Work out the finished part from the listing and answer in its coordinate system (mm). Face numbers are marked on the shaded views. A direction names the side the tool comes from. Coordinates: 2 decimals unless noted, no trailing zeros. Order: outer loops, then holes, each group sorted by start corner. A loop starts at its lowest first (then second) coordinate and runs counter-clockwise, first axis right, second up. Notation, with made-up numbers: M 14,-14 L 32,-14 A16 cw 32,-8 Z; hole C 80.5,36.25 d4. An arc over 180 degrees is marked long. Use a Markdown table: item, result.
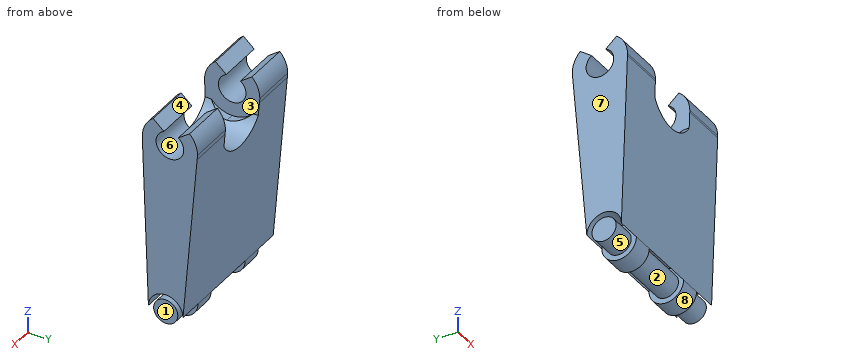
from build123d import *

# Parameters (mm, degrees)
SKETCH1_R           = 4
SKETCH1_R_2         = 5
SKETCH1_R_3         = 3.5
BOSS_EXTRUDE1_DEPTH = 21
SKETCH1_4_R         = 4
CUT_EXTRUDE2_DEPTH  = 8
SKETCH1_5_R         = 5
SKETCH1_5_R_2       = 3.5
CUT_EXTRUDE3_DEPTH  = 8
CUT_EXTRUDE4_START  = 21
SKETCH1_6_R         = 5
SKETCH1_6_R_2       = 3.5
CUT_EXTRUDE4_DEPTH  = 7
CUT_EXTRUDE5_DEPTH  = 10
CUT_EXTRUDE6_REACH  = 71.663


with BuildPart() as part:
    # Sketch1 → Boss-Extrude1 (new, symmetric)
    # profile 1 of 4: a face of its own
    with BuildSketch(Plane(origin=(0, 0, 0), x_dir=(0, 0, -1), z_dir=(1, 0, 0))):
        with BuildLine():
            Line((50, 3.790245356), (1.337639211, 7.887377342))
            ThreePointArc((1.337639211, 7.887377342), (6.111510193, 5.162309866), (8, 0))
            ThreePointArc((8, 0), (5.855645149, -5.450818277), (0.572145029, -7.9795144))
            Line((0.572145029, -7.9795144), (50, -6.209754644))
            ThreePointArc((50, -6.209754644), (45, -1.209754644), (50, 3.790245356))
        make_face()
    # profile 2 of 4: a face of its own
    with BuildSketch(Plane(origin=(0, 0, 0), x_dir=(0, 0, -1), z_dir=(1, 0, 0))):
        with BuildLine():
            Line((1.337639211, 7.887377342), (0, 8))
            ThreePointArc((0, 8), (-8, 0), (0, -8))
            Line((0, -8), (0.572145029, -7.9795144))
            ThreePointArc((0.572145029, -7.9795144), (5.855645149, -5.450818277), (8, 0))
            ThreePointArc((8, 0), (6.111510193, 5.162309866), (1.337639211, 7.887377342))
        make_face()
        with Locations(Location((0, 0, 0), (0, 0, 180))):
            Circle(SKETCH1_R, mode=Mode.SUBTRACT)
    # profile 3 of 4: a face of its own
    with BuildSketch(Plane(origin=(0, 0, 0), x_dir=(0, 0, -1), z_dir=(1, 0, 0))):
        with Locations((50, -1.209754644)):
            Circle(SKETCH1_R_2)
        with Locations((50, -1.209754644)):
            Circle(SKETCH1_R_3, mode=Mode.SUBTRACT)
    # profile 4 of 4: a face of its own
    with BuildSketch(Plane(origin=(0, 0, 0), x_dir=(0, 0, -1), z_dir=(1, 0, 0))):
        with Locations((50, -1.209754644)):
            Circle(SKETCH1_R_3)
    extrude(amount=BOSS_EXTRUDE1_DEPTH, both=True)

    # Sketch1<4> → Cut-Extrude2 (cut, symmetric)
    with BuildSketch(Plane(origin=(0, 0, 0), x_dir=(0, 0, -1), z_dir=(1, 0, 0))):
        with BuildLine():
            Line((1.337639211, 7.887377342), (0, 8))
            ThreePointArc((0, 8), (-8, 0), (0, -8))
            Line((0, -8), (0.572145029, -7.9795144))
            ThreePointArc((0.572145029, -7.9795144), (5.855645149, -5.450818277), (8, 0))
            ThreePointArc((8, 0), (6.111510193, 5.162309866), (1.337639211, 7.887377342))
        make_face()
        with Locations(Location((0, 0, 0), (0, 0, 180))):
            Circle(SKETCH1_4_R, mode=Mode.SUBTRACT)
    extrude(amount=CUT_EXTRUDE2_DEPTH, both=True, mode=Mode.SUBTRACT)

    # Sketch1<5> → Cut-Extrude3 (cut, symmetric)
    with BuildSketch(Plane(origin=(0, 0, 0), x_dir=(0, 0, -1), z_dir=(1, 0, 0))):
        with Locations((50, -1.209754644)):
            Circle(SKETCH1_5_R)
        with Locations((50, -1.209754644)):
            Circle(SKETCH1_5_R_2, mode=Mode.SUBTRACT)
    extrude(amount=CUT_EXTRUDE3_DEPTH, both=True, mode=Mode.SUBTRACT)

    # Sketch1<6> → Cut-Extrude4 (cut)
    with BuildSketch(Plane(origin=(0, 0, 0), x_dir=(0, 0, -1), z_dir=(1, 0, 0)).offset(CUT_EXTRUDE4_START)):
        with Locations((50, -1.209754644)):
            Circle(SKETCH1_6_R)
        with Locations((50, -1.209754644)):
            Circle(SKETCH1_6_R_2, mode=Mode.SUBTRACT)
    cut_extrude4 = extrude(amount=-CUT_EXTRUDE4_DEPTH, mode=Mode.SUBTRACT)

    # Mirror1: Cut-Extrude4 across plane
    add(cut_extrude4.mirror(Plane(origin=(0, 0, 0), x_dir=(0, 0, 1), z_dir=(1, 0, 0))), mode=Mode.SUBTRACT)

    # Sketch3 → Cut-Extrude5 (cut, symmetric)
    with BuildSketch(Plane(origin=(0, 0, 0), x_dir=(1, 0, 0), z_dir=(0, 1, 0))):
        with BuildLine():
            Line((-8, 5.272211447), (-8, -3.420978971))
            Line((-8, -3.420978971), (8, -3.420978971))
            Line((8, -3.420978971), (8, 5.208098852))
            ThreePointArc((8, 5.208098852), (0.018739109, 9.916704947), (-8, 5.272211447))
        make_face()
    extrude(amount=CUT_EXTRUDE5_DEPTH, both=True, mode=Mode.SUBTRACT)

    # Cut-Extrude6: up to this face of the body (flat: up to its plane)
    cut_extrude6_end = Plane(part.part.faces().sort_by_distance((-21, -0.477188429, -19.332209002))[0])
    # Sketch4 → Cut-Extrude6 (cut, up to the picked face)
    with BuildSketch(Plane(origin=(21, 0, 0), x_dir=(0, 0, -1), z_dir=(1, 0, 0)), mode=Mode.PRIVATE) as cut_extrude6_sk1:
        with BuildLine():
            Line((-5.612672438, 5.700693652), (-3.179432131, 2.427181766))
            ThreePointArc((-3.179432131, 2.427181766), (-3.978246032, 0.416603538), (-3.613291572, -1.715844985))
            Line((-3.613291572, -1.715844985), (-6.359318362, -4.853768636))
            ThreePointArc((-6.359318362, -4.853768636), (-7.980056984, 0.564526819), (-5.612672438, 5.700693652))
        make_face()
    cut_extrude6_tool1 = split(extrude(cut_extrude6_sk1.sketch, amount=-CUT_EXTRUDE6_REACH, mode=Mode.PRIVATE), bisect_by=cut_extrude6_end, keep=Keep.BOTH, mode=Mode.PRIVATE)
    add(cut_extrude6_tool1.solids().sort_by(Axis((21, 0.46282, 5.810666), (-1, 0, 0)))[0], mode=Mode.SUBTRACT)


solid = part.part
(1) Determine the mould class of the marked faces 6, 7 and 8 for opening direction Y: pulls with the +Y half, pulls with the -Y half, needs draft (parallel to the pull), parting line crosses it, or undercut.
Conclusion:
| item | result |
|---|---|
| face 6 | undercut |
| face 7 | needs draft |
| face 8 | parting line crosses it |
(2) Which of the six approach directions +Z, -Z, +X, -X, +Y, -Y give full straight-line access (tool end or side, diameter ignored) to the marked faces 1, 2, 3, 4 and 5?
Conclusion:
| item | result |
|---|---|
| face 1 | +Z, -Z, +X, +Y, -Y |
| face 2 | none |
| face 3 | +Z |
| face 4 | +Z, +X, -X |
| face 5 | -X |
(3) A cutting plane is placed at D-D (x = -16.5). Determine the outline of the cut face in (y, z).
Conclusion:
| item | result |
|---|---|
| outline | M -8,0 L -6.21,-50 A5 cw 3.79,-50 L 8,0 A8 ccw 5.7,5.61 L 2.43,3.18 A4 cw long -1.72,3.61 L -4.85,6.36 A8 ccw Z; C -1.21,-50 d7 |
(4) Straight lines are drawn through the part: L1, parallel to X at y = 6, z = -3.5; L2, parallel to Z at x = 16, y = 0; L3, parallel to X at y = 2.5, z = -8.5. For each, find the intervals that lie inside material, in ascending order.
Conclusion:
| item | result |
|---|---|
| L1 | -21 to -8, 8 to 21 |
| L2 | -53.28 to -46.72, -45.15 to -4 |
| L3 | -21 to -4.92, 4.88 to 21 |
(5) Given P1, Ø12, axis at x = -5.5, z = -48, coming from the +Y side; P2, Ø9, axis at y = 0, z = 0, coming from the -X side; P3, Ø2, axis at x = 1.5, z = -33, coming from the -Y side; P4, Ø1.5, axis at x = 7.5, y = -2.5, coming from the -Z side, each flat-ended and moving along its own axis, determine where each tip first touches the part or whether it passes through.
Conclusion:
| item | result |
|---|---|
| P1 | y = 4.46 |
| P2 | x = -21 |
| P3 | y = -6.85 |
| P4 | z = -54.95 |
(6) A cutting plane is placed at A-A (z = -6). Determine the outline of the cut face in (x, y), then the cut area to 3 significant figures.
Conclusion:
| item | result |
|---|---|
| outline | M -21,-7.79 L -7.54,-7.79 L -7.54,-5.29 L -8,-5.29 L -8,5.29 L -7.54,5.29 L -7.54,7.49 L -21,7.49 Z; M 7.5,-7.79 L 21,-7.79 L 21,7.49 L 7.5,7.49 L 7.5,5.29 L 8,5.29 L 8,-5.29 L 7.5,-5.29 Z |
| area | 402 mm2 |
(7) A cutting plane is placed at B-B (x = -1). Determine the outline of the cut face in (y, z).
Conclusion:
| item | result |
|---|---|
| outline | M -7.65,-9.86 L -6.21,-50 A5 cw 3.79,-50 L 7.17,-9.86 Z; C -1.21,-50 d7 |
(8) A cutting plane is placed at C-C (y = 4.75). Determine the outline of the cut face in (x, z).
Conclusion:
| item | result |
|---|---|
| outline | M -21,-38.6 L 21,-38.6 L 21,4.91 L 8,4.91 L 8,-6.44 L 7.18,-6.44 A9.18 cw -7.21,-6.44 L -8,-6.44 L -8,4.91 L -21,4.91 Z |
